Here's how the part is built. I have some questions about the finished solid (model axes, mm). Coordinates: 2 decimals unless noted, no trailing zeros. Loops run counter-clockwise (first coordinate to the right, second up) from the corner with the lowest first, then second, coordinate; pieces in that order, holes last. Notation, with made-up numbers: (40.5, -8.5) -> (79.5, -8.5) arc R13 cw to (79.5, 0.5) -> close; hole circle Ø6 at (69, -18.75). An arc over 180 degrees is marked (long way). Answer as a JSON object with one key per item and string values. Group by question number.
1) I want a section at A-A (y = 0). Write out the boundary of the cut face in (x, z), then the cut area to 3 significant figures.
2) If we mould it in two halves opening along X, with no side actions, what happens to faces 1 (the flat face through (0, -4, 0)), 2 (the cylindrical face through (8.584, 2.703, 10.846)), 3 (the cylindrical face through (-3, 0, 11))? For each: +X half, -X half, draft (parallel to the pull), parting line (faces both ways), or undercut.
3) I want a section at C-C (z = 17). Write out the boundary of the cut face in (x, y), then the cut area to 3 significant figures.
4) I'm going to push flat-ended pins straight in: pin 1 (6 mm diameter, centred on x = -6.5, z = 3, fed in from -Y); pin 2 (3 mm diameter, centred on y = 6, z = 18.5, fed in from +X); pin 3 (5 mm diameter, centred on x = 7, z = 11, fed in from +Y); pin 4 (5.5 mm diameter, centred on x = 0, y = 0, fed in from -Z). Where does each tip first touch, or does it pass through?
5) I want a section at B-B (x = 0). Write out the boundary of the cut face in (y, z).
6) I need wall thicknesses on probe 1 along Z at (x, y) = (7, 0); probe 2 along Y at (x, z) = (0, 12.25); probe 3 along Z at (x, y) = (-7, -0.75). Which ranges of each line are inside material? Lowest first, please. Write a range as [from, to].
7) I want a section at D-D (z = 19.75). Write out the boundary of the cut face in (x, y).
```python
from build123d import *

# Parameters (mm, degrees)
F0_R          = 9
F0_R_2        = 3
F1_DEPTH      = 22
F2_R          = 1.75
F3_DEPTH      = 9.001
F3_DEPTH_BACK = 25


with BuildPart() as f1:
    # F0 (on Top) → F1 (new body)
    with BuildSketch(Plane.XY):
        Circle(F0_R)
        Circle(F0_R_2, mode=Mode.SUBTRACT)
    extrude(amount=F1_DEPTH)

    # F2 (on Right) → F3 (cut, two sides)
    with BuildSketch(Plane.YZ) as f3_sk:
        with Locations((0, 5)):
            Circle(F2_R)
        with Locations((0, 17)):
            Circle(F2_R)
    extrude(amount=-F3_DEPTH, mode=Mode.SUBTRACT)
    extrude(f3_sk.sketch, amount=F3_DEPTH_BACK, mode=Mode.SUBTRACT)


solid = f1.part
```
Determined:
{
 "1": {"outline": "(-9, 0) -> (-3, 0) -> (-3, 3.25) -> (-9, 3.25) -> close; (-9, 6.75) -> (-3, 6.75) -> (-3, 15.25) -> (-9, 15.25) -> close; (-9, 18.75) -> (-3, 18.75) -> (-3, 22) -> (-9, 22) -> close; (3, 0) -> (9, 0) -> (9, 3.25) -> (3, 3.25) -> close; (3, 6.75) -> (9, 6.75) -> (9, 15.25) -> (3, 15.25) -> close; (3, 18.75) -> (9, 18.75) -> (9, 22) -> (3, 22) -> close", "area": "180 mm^2"},
 "2": {"face 1": "draft", "face 2": "parting line", "face 3": "undercut"},
 "3": {"outline": "(-8.83, -1.75) arc R9 ccw to (8.83, -1.75) -> (2.44, -1.75) arc R3 cw to (-2.44, -1.75) -> close; (-8.83, 1.75) -> (-2.44, 1.75) arc R3 cw to (2.44, 1.75) -> (8.83, 1.75) arc R9 ccw to start", "area": "183 mm^2"},
 "4": {"pin 1": "y = -8.29", "pin 2": "x = 7.79", "pin 3": "y = 7.79", "pin 4": "through"},
 "5": {"outline": "(-9, 0) -> (-3, 0) -> (-3, 22) -> (-9, 22) -> close; (3, 0) -> (9, 0) -> (9, 22) -> (3, 22) -> close"},
 "6": {"probe 1": "[0, 3.25], [6.75, 15.25], [18.75, 22]", "probe 2": "[-9, -3], [3, 9]", "probe 3": "[0, 3.42], [6.58, 15.42], [18.58, 22]"},
 "7": {"outline": "circle Ø18 at (0, 0); hole circle Ø6 at (0, 0)"}
}
